```python
from build123d import *

# Parameters (mm, degrees)
TAPPED_HOLE_FOR_9_16_12_HELICOIL1_D = 14.68374


with BuildPart() as part:
    # Sketch1 → Revolve2 (revolve)
    with BuildSketch(Plane(origin=(0, 0, 0), x_dir=(1, 0, 0), z_dir=(0, 1, 0))):
        Polygon((929.772285353, 97.830519041), (929.772285353, 76.2), (948.822285353, 76.2), (948.822285353, 94.885801773), align=None)
    revolve(axis=Axis((1049.721128595, 0, -76.2), (-1, 0, 0)))

    # Tapped Hole for 9/16-12 Helicoil1 (through all)
    with Locations(Plane.ZY.offset(-929.772285353)):
        with Locations((-76.2, 0)):
            Hole(TAPPED_HOLE_FOR_9_16_12_HELICOIL1_D / 2)

    # Sketch5 → Cut-Revolve1 (revolve, cut)
    with BuildSketch(Plane(origin=(0, 0, 0), x_dir=(1, 0, 0), z_dir=(0, 1, 0))):
        with BuildLine():
            Line((927.609152682, 95.594725662), (927.609152682, 86.08187))
            Line((927.609152682, 86.08187), (943.107285353, 86.08187))
            ThreePointArc((943.107285353, 86.08187), (945.352349383, 87.01180597), (946.282285353, 89.25687))
            Line((946.282285353, 89.25687), (946.282285353, 89.986341597))
            ThreePointArc((946.282285353, 89.986341597), (945.517739835, 92.052820291), (943.592311059, 93.124075663))
            Line((943.592311059, 93.124075663), (927.609152682, 95.594725662))
        make_face()
    revolve(axis=Axis((1049.721128595, 0, -76.2), (-1, 0, 0)), mode=Mode.SUBTRACT)


solid = part.part
```
Input: part model. Units: mm. Frame: model coordinates. A direction names the side the tool comes from. Give positions to 0.01 mm unless a question says otherwise; leave off trailing zeros. Order: outer loops, then holes, each group sorted by start corner. A loop starts at its lowest first (then second) coordinate and runs counter-clockwise, first axis right, second up. Notation, with made-up numbers: (-21, 38) -> (27, 38) arc R30 cw to (27, 65) -> close; hole circle Ø9 at (21, 84.25). An arc over 180 degrees is marked (long way). Write each question's results on one line, items separated by ' | '. Start each with the question number.
Item 1: Set-up query: faces 4 (the flat face through (946.282, 7, -65)), 5 (the cylindrical face through (939.43, 2.21, -83.2)). Return all of +Z, -Z, +X, -X, +Y, -Y with unobstructed straight access to the full face (end or side cutting, diameter ignored); none if empty.
Item 2: Cut plane B-B on y = 0. Return the cut outline in (x, z) (3 decimals), then the cut area to 3 significant figures.
Item 3: Contact query for flat-ended pins moving along their axis: P1, Ø10, axis at x = 938, z = -78.5, coming from the +Y side; P2, Ø3, axis at x = 938, z = -63, coming from the -Y side; P3, Ø4, axis at x = 937.5, z = -77, coming from the -Y side. Output: stop coordinate, or through.
Item 4: Cut plane C-C on x = 934. Return the cut outline in (y, z), then the cut area to 3 significant figures.
Item 5: Cut plane D-D on x = 938.75. Return the cut outline in (y, z), then the cut area to 3 significant figures.
Item 6: Mould query, pull axis Y, two halves, no side actions, for faces 1 (the flat face through (929.772, 18, -84)), 2 (the cylindrical face through (936.533, -2.968, -85.626)), 3 (the conical face through (941.281, -0.873, -56.368)). Classes: pulls with the +Y half, pulls with the -Y half, needs draft (parallel to the pull), parting line crosses it, or undercut.
Item 7: Cut plane A-A on z = -76.2. Return the cut outline in (x, y) (3 decimals).
Item 8: Line query: line 1 (Y direction, x = 942.5, z = -76.2); line 2 (Z direction, x = 938.25, y = 2); line 3 (Z direction, x = 945, y = 3). Output: solid intervals per line, ascending.
Established:
1) face 4: -X | face 5: +X, -X
2) outline: (929.772, -97.831) -> (948.822, -94.886) -> (948.822, -83.542) -> (929.772, -83.542) -> (929.772, -86.082) -> (943.107, -86.082) arc R3.175 cw to (946.282, -89.257) -> (946.282, -89.986) arc R3.175 cw to (943.592, -93.124) -> (929.772, -95.26) -> close; (929.772, -68.858) -> (948.822, -68.858) -> (948.822, -57.514) -> (929.772, -54.569) -> (929.772, -57.14) -> (943.592, -59.276) arc R3.175 cw to (946.282, -62.414) -> (946.282, -63.143) arc R3.175 cw to (943.107, -66.318) -> (929.772, -66.318) -> close | area: 235 mm^2
3) P1: y = 21.08 | P2: y = -16.7 | P3: y = -20.74
4) outline: circle Ø41.95 at (0, -76.2); circle Ø19.76 at (0, -76.2); hole circle Ø36.81 at (0, -76.2); hole circle Ø14.68 at (0, -76.2) | area: 455 mm^2
5) outline: circle Ø40.49 at (0, -76.2); circle Ø19.76 at (0, -76.2); hole circle Ø35.35 at (0, -76.2); hole circle Ø14.68 at (0, -76.2) | area: 444 mm^2
6) face 1: needs draft | face 2: undercut | face 3: parting line crosses it
7) outline: (929.772, -21.631) -> (948.822, -18.686) -> (948.822, -7.342) -> (929.772, -7.342) -> (929.772, -9.882) -> (943.107, -9.882) arc R3.175 cw to (946.282, -13.057) -> (946.282, -13.786) arc R3.175 cw to (943.592, -16.924) -> (929.772, -19.06) -> close; (929.772, 7.342) -> (948.822, 7.342) -> (948.822, 18.686) -> (929.772, 21.631) -> (929.772, 19.06) -> (943.592, 16.924) arc R3.175 cw to (946.282, 13.786) -> (946.282, 13.057) arc R3.175 cw to (943.107, 9.882) -> (929.772, 9.882) -> close
8) line 1: -19.66 to -17.09, -9.88 to -7.34, 7.34 to 9.88, 17.09 to 19.66 | line 2: -96.42 to -93.84, -85.88 to -83.26, -69.14 to -66.52, -58.56 to -55.98 | line 3: -95.24 to -92.26, -86.27 to -82.9, -69.5 to -66.13, -60.14 to -57.16
